Verification items for the finished model (mm, model axes). Face numbers are marked on the shaded views. Coordinates: 2 decimals unless noted, no trailing zeros. Use one line per item in the form item = value. Start each with the question number.
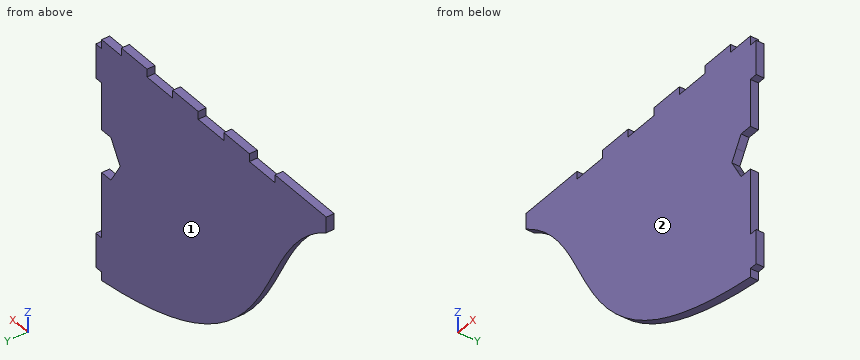
```python
from build123d import *

# Parameters (mm, degrees)
F0_W      = 279.4
F0_H      = 330.2
F1_DEPTH  = 5.842
F2_W      = 25.4
F2_H      = 5.842
F2_W_2    = 76.2
F2_W_3    = 5.842
F2_H_2    = 25.4
F2_H_3    = 38.1
F3_DEPTH  = 5.842
F5_W      = 5.842
F5_H      = 12.7
F6_DEPTH  = 5.842
F7_DEPTH  = 5.842
F8_W      = 5.842
F8_H      = 48.641
F8_H_2    = 34.925
F8_H_3    = 11.684
F9_DEPTH  = 5.842
F10_W     = 246.7240431406
F10_H     = 1.016
F11_DEPTH = 5.842
F12_W     = 25.4
F12_H     = 5.842
F12_W_2   = 19.558
F13_DEPTH = 5.842


with BuildPart() as f1:
    # F0 (on Front) → F1 (new body)
    with BuildSketch(Plane.XZ):
        with Locations((25.751306051, 40.8756073241)):
            Rectangle(F0_W, F0_H)
    extrude(amount=F1_DEPTH)

    # F2 (on face) → F3 (cut, through all)
    with BuildSketch(Plane.XZ.offset(5.842)):
        with Locations((152.751306051, -121.3033926759)):
            Rectangle(F2_W, F2_H)
        with Locations((101.951306051, -121.3033926759)):
            Rectangle(F2_W, F2_H)
        with Locations((51.151306051, -121.3033926759)):
            Rectangle(F2_W, F2_H)
        with Locations((0.351306051, -121.3033926759)):
            Rectangle(F2_W, F2_H)
        with Locations((-75.848693949, -121.3033926759)):
            Rectangle(F2_W_2, F2_H)
        with Locations((162.530306051, -86.1243926759)):
            Rectangle(F2_W_3, F2_H_2)
        with Locations((162.530306051, -28.9743926759)):
            Rectangle(F2_W_3, F2_H_3)
        with Locations((-111.027693949, -86.1243926759)):
            Rectangle(F2_W_3, F2_H_2)
        with Locations((-111.027693949, -35.3243926759)):
            Rectangle(F2_W_3, F2_H_2)
        with Locations((-111.027693949, 15.4756073241)):
            Rectangle(F2_W_3, F2_H_2)
        with Locations((-111.027693949, 66.2756073241)):
            Rectangle(F2_W_3, F2_H_2)
        with Locations((-111.027693949, 167.8756073241)):
            Rectangle(F2_W_3, F2_H_2)
        with Locations((-111.027693949, 117.0756073241)):
            Rectangle(F2_W_3, F2_H_2)
    extrude(amount=-F3_DEPTH, mode=Mode.SUBTRACT)

    # F5 (on face) → F6 (cut, through all)
    with BuildSketch(Plane.XZ.offset(5.842)):
        with Locations((162.530306051, 2.7756073241)):
            Rectangle(F5_W, F5_H)
    extrude(amount=-F6_DEPTH, mode=Mode.SUBTRACT)

    # F4 (on face) → F7 (cut, through all)
    with BuildSketch(Plane.XZ.offset(5.842)):
        with BuildLine():
            Line((165.451306051, 15.4756073241), (159.609306051, 15.4756073241))
            add(Edge.make_bspline(
                [(159.609306051, 15.4756073241), (73.376306051, 28.1756073241), (-24.3765935073, 60.3637718481), (-21.873693949, 193.2756073241), (-113.948693949, 205.9756073241)],
                knots=[0, 0, 0, 0, 0.507272, 1, 1, 1, 1], degree=3))
            Line((-113.948693949, 205.9756073241), (-113.948693949, 180.5756073241))
            Line((-113.948693949, 180.5756073241), (-108.106693949, 180.5756073241))
            Line((-108.106693949, 180.5756073241), (-108.106693949, 155.1756073241))
            Line((-108.106693949, 155.1756073241), (-113.948693949, 155.1756073241))
            Line((-113.948693949, 155.1756073241), (-113.948693949, 129.7756073241))
            Line((-113.948693949, 129.7756073241), (-108.106693949, 129.7756073241))
            Line((-108.106693949, 129.7756073241), (-108.106693949, 104.3756073241))
            Line((-108.106693949, 104.3756073241), (-113.948693949, 104.3756073241))
            Line((-113.948693949, 104.3756073241), (-113.948693949, 78.9756073241))
            Line((-113.948693949, 78.9756073241), (-108.106693949, 78.9756073241))
            Line((-108.106693949, 78.9756073241), (-108.106693949, 53.5756073241))
            Line((-108.106693949, 53.5756073241), (-113.948693949, 53.5756073241))
            Line((-113.948693949, 53.5756073241), (-113.948693949, 28.1756073241))
            Line((-113.948693949, 28.1756073241), (-108.106693949, 28.1756073241))
            Line((-108.106693949, 28.1756073241), (-108.106693949, 2.7756073241))
            Line((-108.106693949, 2.7756073241), (-113.948693949, 2.7756073241))
            Line((-113.948693949, 2.7756073241), (-113.948693949, -22.6243926759))
            Line((-113.948693949, -22.6243926759), (-108.106693949, -22.6243926759))
            Line((-108.106693949, -22.6243926759), (-108.106693949, -48.0243926759))
            Line((-108.106693949, -48.0243926759), (-113.948693949, -48.0243926759))
            Line((-113.948693949, -48.0243926759), (-113.948693949, -73.4243926759))
            Line((-113.948693949, -73.4243926759), (-108.106693949, -73.4243926759))
            Line((-108.106693949, -73.4243926759), (-108.106693949, -98.8243926759))
            Line((-108.106693949, -98.8243926759), (-113.948693949, -98.8243926759))
            Line((-113.948693949, -98.8243926759), (-113.948693949, -118.3823926759))
            Line((-113.948693949, -118.3823926759), (-37.748693949, -118.3823926759))
            Line((-37.748693949, -118.3823926759), (-37.748693949, -124.2243926759))
            Line((-37.748693949, -124.2243926759), (-12.348693949, -124.2243926759))
            Line((-12.348693949, -124.2243926759), (-12.348693949, -118.3823926759))
            Line((-12.348693949, -118.3823926759), (13.051306051, -118.3823926759))
            Line((13.051306051, -118.3823926759), (13.051306051, -124.2243926759))
            Line((13.051306051, -124.2243926759), (38.451306051, -124.2243926759))
            Line((38.451306051, -124.2243926759), (38.451306051, -118.3823926759))
            Line((38.451306051, -118.3823926759), (63.851306051, -118.3823926759))
            Line((63.851306051, -118.3823926759), (63.851306051, -124.2243926759))
            Line((63.851306051, -124.2243926759), (89.251306051, -124.2243926759))
            Line((89.251306051, -124.2243926759), (89.251306051, -118.3823926759))
            Line((89.251306051, -118.3823926759), (114.651306051, -118.3823926759))
            Line((114.651306051, -118.3823926759), (114.651306051, -124.2243926759))
            Line((114.651306051, -124.2243926759), (140.051306051, -124.2243926759))
            Line((140.051306051, -124.2243926759), (140.051306051, -118.3823926759))
            Line((140.051306051, -118.3823926759), (165.451306051, -118.3823926759))
            Line((165.451306051, -118.3823926759), (165.451306051, -98.8243926759))
            Line((165.451306051, -98.8243926759), (159.609306051, -98.8243926759))
            Line((159.609306051, -98.8243926759), (159.609306051, -73.4243926759))
            Line((159.609306051, -73.4243926759), (165.451306051, -73.4243926759))
            Line((165.451306051, -73.4243926759), (165.451306051, -48.0243926759))
            Line((165.451306051, -48.0243926759), (159.609306051, -48.0243926759))
            Line((159.609306051, -48.0243926759), (159.609306051, -9.9243926759))
            Line((159.609306051, -9.9243926759), (165.451306051, -9.9243926759))
            Line((165.451306051, -9.9243926759), (165.451306051, 15.4756073241))
        make_face()
        with BuildLine():
            add(Edge.make_bspline(
                [(159.609306051, 15.4756073241), (73.376306051, 28.1756073241), (-24.3765935073, 60.3637718481), (-21.873693949, 193.2756073241), (-113.948693949, 205.9756073241)],
                knots=[0, 0, 0, 0, 0.507272, 1, 1, 1, 1], degree=3))
            Line((159.609306051, 15.4756073241), (159.609306051, 21.8256073241))
            add(Edge.make_bspline(
                [(159.609306051, 21.8256073241), (63.851306051, 34.5256073241), (-5.6173037023, 95.4914607938), (-31.4644745687, 187.7697107475), (-87.114737086, 205.9756073241)],
                knots=[0, 0, 0, 0, 0.5236819738, 0.940243193, 0.940243193, 0.940243193, 0.940243193], degree=3))
            Line((-87.114737086, 205.9756073241), (-113.948693949, 205.9756073241))
        make_face()
    extrude(amount=-F7_DEPTH, mode=Mode.SUBTRACT)

    # F8 (on face) → F9 (cut, through all)
    with BuildSketch(Plane.XZ.offset(5.842)):
        Polygon((165.451306051, 15.4756073241), (165.451306051, 28.1756073241), (159.609306051, 28.1756073241), (159.609306051, 21.8256073241), (159.609306051, 15.4756073241), align=None)
        with Locations((162.530306051, 77.8961073241)):
            Rectangle(F8_W, F8_H)
        with BuildLine():
            Line((159.609306051, 102.2166073241), (165.451306051, 102.2166073241))
            Line((165.451306051, 102.2166073241), (165.451306051, 103.3306229057))
            ThreePointArc((165.451306051, 103.3306229057), (162.5829399691, 102.4975980153), (159.609306051, 102.2166073241))
        make_face()
        with BuildLine():
            ThreePointArc((145.861152343, 110.1541080567), (151.6718056847, 104.3434542505), (159.609306051, 102.2166073241))
            Line((159.609306051, 102.2166073241), (159.609306051, 133.9666073241))
            ThreePointArc((159.609306051, 133.9666073241), (151.6718056847, 131.8397603977), (145.861152343, 126.0291065915))
            ThreePointArc((145.861152343, 126.0291065915), (143.734306051, 118.0916073241), (145.861152343, 110.1541080567))
        make_face()
        with BuildLine():
            Line((150.4438705276, 102.2166073241), (159.609306051, 102.2166073241))
            ThreePointArc((159.609306051, 102.2166073241), (151.6718056847, 104.3434542505), (145.861152343, 110.1541080567))
            Line((145.861152343, 110.1541080567), (150.4438705276, 102.2166073241))
        make_face()
        with BuildLine():
            Line((159.609306051, 133.9666073241), (159.609306051, 102.2166073241))
            ThreePointArc((159.609306051, 102.2166073241), (162.5829399691, 102.4975980153), (165.451306051, 103.3306229057))
            Line((165.451306051, 103.3306229057), (165.451306051, 132.8525917425))
            ThreePointArc((165.451306051, 132.8525917425), (162.5829399691, 133.6856166328), (159.609306051, 133.9666073241))
        make_face()
        with BuildLine():
            Line((165.451306051, 133.9666073241), (159.609306051, 133.9666073241))
            ThreePointArc((159.609306051, 133.9666073241), (162.5829399691, 133.6856166328), (165.451306051, 132.8525917425))
            Line((165.451306051, 132.8525917425), (165.451306051, 133.9666073241))
        make_face()
        with BuildLine():
            ThreePointArc((145.861152343, 126.0291065915), (151.6718056847, 131.8397603977), (159.609306051, 133.9666073241))
            Line((159.609306051, 133.9666073241), (150.4438705276, 133.9666073241))
            Line((150.4438705276, 133.9666073241), (145.861152343, 126.0291065915))
        make_face()
        with Locations((162.530306051, 151.4291073241)):
            Rectangle(F8_W, F8_H_2)
        with BuildLine():
            Line((141.2784350042, 118.0916073241), (145.861152343, 110.1541080567))
            ThreePointArc((145.861152343, 110.1541080567), (143.734306051, 118.0916073241), (145.861152343, 126.0291065915))
            Line((145.861152343, 126.0291065915), (141.2784350042, 118.0916073241))
        make_face()
        with Locations((162.530306051, 200.1336073241)):
            Rectangle(F8_W, F8_H_3)
    extrude(amount=-F9_DEPTH, mode=Mode.SUBTRACT)

    # F10 (on face) → F11 (join, through all)
    with BuildSketch(Plane.XZ.offset(5.842)):
        with Locations((36.2472844807, 206.4836073241)):
            Rectangle(F10_W, F10_H)
    extrude(amount=-F11_DEPTH)

    # F12 (on face) → F13 (cut, through all)
    with BuildSketch(Plane.XZ.offset(5.842)):
        with Locations((51.151306051, 204.0706073241)):
            Rectangle(F12_W, F12_H)
        with Locations((101.951306051, 204.0706073241)):
            Rectangle(F12_W, F12_H)
        with Locations((149.830306051, 204.0706073241)):
            Rectangle(F12_W_2, F12_H)
        with BuildLine():
            add(Edge.make_bspline(
                [(-64.0656111495, 195.8912068503), (-64.4986133811, 197.8821506555), (-64.5462177809, 200.9608220943), (-64.8897370896, 206.9916073241)],
                knots=[0.7783755915, 0.7783755915, 0.7783755915, 0.7783755915, 1, 1, 1, 1], degree=3))
            Line((-64.8897370896, 206.9916073241), (-87.1147370896, 206.9916073241))
            Line((-87.1147370896, 206.9916073241), (-87.1147370896, 205.9756073241))
            add(Edge.make_bspline(
                [(-64.0656111419, 195.8912068549), (-70.8038372609, 199.7329606353), (-78.4197996839, 203.1310721158), (-87.114737086, 205.9756073241)],
                knots=[0.8751586172, 0.8751586172, 0.8751586172, 0.8751586172, 0.940243193, 0.940243193, 0.940243193, 0.940243193], degree=3))
        make_face()
        with Locations((0.351306051, 204.0706073241)):
            Rectangle(F12_W, F12_H)
        with BuildLine():
            Line((-63.148693949, 195.362557311), (-63.148693949, 206.9916073241))
            Line((-63.148693949, 206.9916073241), (-64.8897370896, 206.9916073241))
            add(Edge.make_bspline(
                [(-64.0656111495, 195.8912068503), (-64.4986133811, 197.8821506555), (-64.5462177809, 200.9608220943), (-64.8897370896, 206.9916073241)],
                knots=[0.7783755915, 0.7783755915, 0.7783755915, 0.7783755915, 1, 1, 1, 1], degree=3))
            add(Edge.make_bspline(
                [(-63.148693949, 195.362557311), (-63.4525182871, 195.5396905387), (-63.7581509788, 195.7159105346), (-64.0656111419, 195.8912068549)],
                knots=[0.8721888572, 0.8721888572, 0.8721888572, 0.8721888572, 0.8751586172, 0.8751586172, 0.8751586172, 0.8751586172], degree=3))
        make_face()
    extrude(amount=-F13_DEPTH, mode=Mode.SUBTRACT)


solid = f1.part
```
1. Release check for a two-part mould opening along Y. For the marked faces 1 and 2 record: pulls with the +Y half, pulls with the -Y half, needs draft (parallel to the pull), parting line crosses it, or undercut.
2. Depth check by flat-ended pin: P1, Ø3, axis at x = 56, y = -3, coming from the +Z side; P2, Ø1, axis at y = -2.5, z = 76.5, coming from the -X side; P3, Ø1.8, axis at y = -4, z = 204, coming from the +X side. Enter the tip coordinate at first touch or a pass-through.
3. Material ranges on line 1 along Z through (x, y) = (142, -2.3); line 2 along X through (y, z) = (-3.65, 49); line 3 along X through (y, z) = (-1.25, 89), recorded low to high.
Final values:
q1.face_1 = pulls with the +Y half
q1.face_2 = pulls with the -Y half
q2.P1 = 201.15
q2.P2 = 26.26
q2.P3 = 140.05
q3.line_1 = 24.51 to 116.84, 119.34 to 201.15
q3.line_2 = 64.43 to 165.45
q3.line_3 = 15.62 to 159.61
